The listing builds one solid part. Answer for the finished solid, in the listing's coordinates (mm). Round coordinates to 2 decimals unless told otherwise and drop trailing zeros. Loops run counter-clockwise (first coordinate to the right, second up) from the corner with the lowest first, then second, coordinate; pieces in that order, holes last. Notation, with made-up numbers: (-19.5, 36.5) - (-13.5, 36.5) arc R10 ccw to (-13.5, 45.5) - close; hole circle Ø1 at (34.25, 67.5). An arc over 180 degrees is marked (long way). One line per item, written item: value.
```python
from build123d import *

# Parameters (mm, degrees)
SKETCH1_W                  = 2.5
SKETCH1_H                  = 8
BOSS_EXTRUDE1_DEPTH        = 2.5
SKETCH2_W                  = 1.5
SKETCH2_H                  = 1.5
CUT_EXTRUDE2_DEPTH         = 7
CHAMFER3_SIZE              = 0.25
LPATTERN2_COUNT            = 10
LPATTERN2_PITCH            = 2.5
CHAMFER3_OF_LPATTERN2_SIZE = 0.25


with BuildPart() as part:
    # Sketch1 → Boss-Extrude1 (new body)
    with BuildSketch(Plane.XY):
        Rectangle(SKETCH1_W, SKETCH1_H)
    boss_extrude1 = extrude(amount=BOSS_EXTRUDE1_DEPTH)

    # Sketch2 → Cut-Extrude2 (cut)
    with BuildSketch(Plane(origin=(0, 4, 0), x_dir=(1, 0, 0), z_dir=(0, 1, 0))):
        with Locations((0, -1.25)):
            Rectangle(SKETCH2_W, SKETCH2_H)
    cut_extrude2 = extrude(amount=-CUT_EXTRUDE2_DEPTH, mode=Mode.SUBTRACT)

    # Chamfer3
    chamfer3_edges = [part.edges().sort_by_distance(p)[0] for p in [
        (0, 4, 2),
        (0.75, 4, 1.25),
        (0, 4, 0.5),
        (-0.75, 4, 1.25),
    ]]
    chamfer(chamfer3_edges, length=CHAMFER3_SIZE)

    # LPattern2: Boss-Extrude1, Cut-Extrude2 ×10
    with Locations(*[(i * LPATTERN2_PITCH, 0, 0) for i in range(1, LPATTERN2_COUNT)]):
        add(boss_extrude1)
        add(cut_extrude2, mode=Mode.SUBTRACT)

    # Chamfer3 of LPattern2
    chamfer3_of_lpattern2_edges = [part.edges().sort_by_distance(p)[0] for p in [
        (2.5, 4, 2),
        (3.25, 4, 1.25),
        (2.5, 4, 0.5),
        (1.75, 4, 1.25),
        (5, 4, 2),
        (5.75, 4, 1.25),
        (5, 4, 0.5),
        (4.25, 4, 1.25),
        (7.5, 4, 2),
        (8.25, 4, 1.25),
        (7.5, 4, 0.5),
        (6.75, 4, 1.25),
        (10, 4, 2),
        (10.75, 4, 1.25),
        (10, 4, 0.5),
        (9.25, 4, 1.25),
        (12.5, 4, 2),
        (13.25, 4, 1.25),
        (12.5, 4, 0.5),
        (11.75, 4, 1.25),
        (15, 4, 2),
        (15.75, 4, 1.25),
        (15, 4, 0.5),
        (14.25, 4, 1.25),
        (17.5, 4, 2),
        (18.25, 4, 1.25),
        (17.5, 4, 0.5),
        (16.75, 4, 1.25),
        (20, 4, 2),
        (20.75, 4, 1.25),
        (20, 4, 0.5),
        (19.25, 4, 1.25),
        (22.5, 4, 2),
        (23.25, 4, 1.25),
        (22.5, 4, 0.5),
        (21.75, 4, 1.25),
    ]]
    chamfer(chamfer3_of_lpattern2_edges, length=CHAMFER3_OF_LPATTERN2_SIZE)


solid = part.part
```
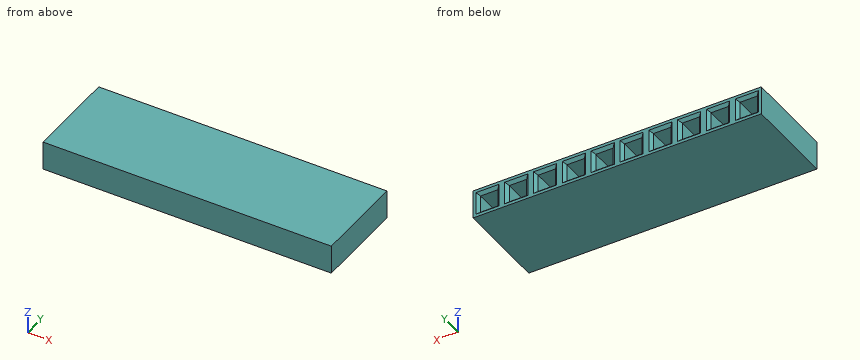
1) A cutting plane is placed at A-A on x = 12.25. Give the vertices of the cut face in (y, z), and give its area (3 significant figures).
Final values:
outline: (-4, 0) - (4, 0) - (4, 0.25) - (3.75, 0.5) - (-3, 0.5) - (-3, 2) - (3.75, 2) - (4, 2.25) - (4, 2.5) - (-4, 2.5) - close
area: 9.44 mm2
2) Consider L1, parallel to Z at x = 3, y = 0.25; L2, parallel to Y at x = 22.5, z = 0.6; L3, parallel to Y at x = 12.75, z = 2.2. Determine where each line is inside the solid, lowest interval first.
Final values:
L1: 0 to 0.5, 2 to 2.5
L2: -4 to -3
L3: -4 to 3.95
3) A cutting plane is placed at B-B on y = -1. Give the number of separate pieces and of enclosed holes in the cut face, and give its area (3 significant figures).
Final values:
separate pieces: 1
enclosed holes: 10
area: 40.0 mm2
4) Each of these flat-tipped pins is pushed along its axis until it touches: pin 1 Ø2 at (x, y) = (6.5, 2) entering from -Z; pin 2 Ø0.8 at (x, z) = (13, 1.5) entering from +Y. Where does it stop, or does it pass through?
Final values:
pin 1: z = 0
pin 2: y = 3.9
